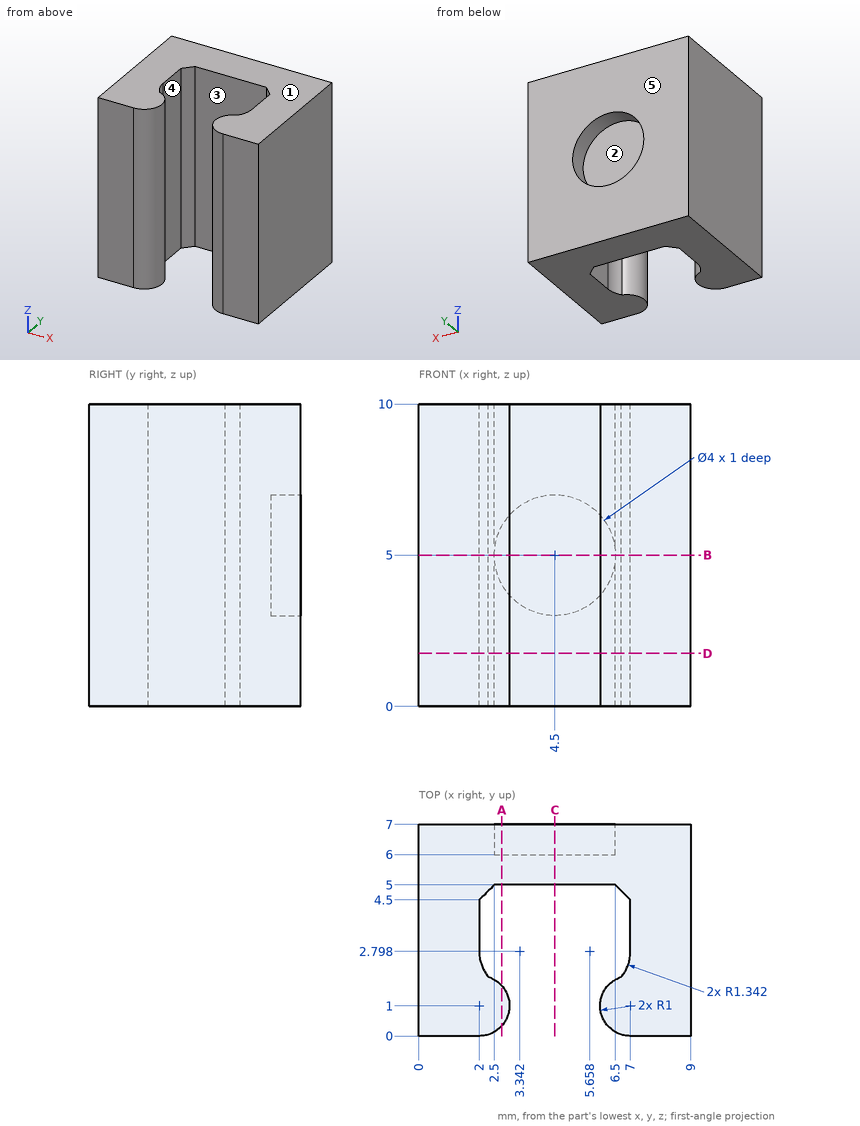
Geometry: see drawing. Coordinates: mm, zero at the bounding-box minimum. A direction names the side the tool comes from. Round coordinates to 2 decimals unless told otherwise and drop trailing zeros. Loops run counter-clockwise (first coordinate to the right, second up) from the corner with the lowest first, then second, coordinate; pieces in that order, holes last. Notation, with made-up numbers: (78.25, 69) -> (103.25, 69) arc R21 cw to (103.25, 74) -> close; hole circle Ø2 at (3, 60). An arc over 180 degrees is marked (long way). Write each question's results on one line, items separated by ' | '.
Item 1: Pull-direction query (Y, two-part tool) for the marked faces 1, 2 and 3; classes: pulls with the +Y half, pulls with the -Y half, needs draft (parallel to the pull), parting line crosses it, or undercut.
Answers below:
face 1: needs draft | face 2: pulls with the +Y half | face 3: undercut
Item 2: Cut plane A-A on x = 2.75. Return the cut outline in (y, z), and give its area (3 significant figures).
Answers below:
outline: (0.34, 0) -> (1.66, 0) -> (1.66, 10) -> (0.34, 10) -> close; (5, 0) -> (7, 0) -> (7, 4.03) -> (6, 4.03) -> (6, 5.97) -> (7, 5.97) -> (7, 10) -> (5, 10) -> close | area: 31.3 mm²
Item 3: Set-up query: the marked faces 4 and 5. Return all of +Z, -Z, +X, -X, +Y, -Y with unobstructed straight access to the full face (end or side cutting, diameter ignored); none if empty.
Answers below:
face 4: +Z, -Z | face 5: +Z, -Z, +X, -X, +Y
Item 4: Cut plane B-B on z = 5. Return the cut outline in (x, y) (1 decimal).
Answers below:
outline: (0, 0) -> (2, 0) arc R1 ccw to (2.3, 2) arc R1.3 cw to (2, 2.8) -> (2, 4.5) -> (2.5, 5) -> (6.5, 5) -> (7, 4.5) -> (7, 2.8) arc R1.3 cw to (6.7, 2) arc R1 ccw to (7, 0) -> (9, 0) -> (9, 7) -> (6.5, 7) -> (6.5, 6) -> (2.5, 6) -> (2.5, 7) -> (0, 7) -> close
Item 5: Cut plane C-C on x = 4.5. Return the cut outline in (y, z).
Answers below:
outline: (5, 0) -> (7, 0) -> (7, 3) -> (6, 3) -> (6, 7) -> (7, 7) -> (7, 10) -> (5, 10) -> close
Item 6: Cut plane D-D on z = 1.75. Return the cut outline in (x, y) (1 decimal).
Answers below:
outline: (0, 0) -> (2, 0) arc R1 ccw to (2.3, 2) arc R1.3 cw to (2, 2.8) -> (2, 4.5) -> (2.5, 5) -> (6.5, 5) -> (7, 4.5) -> (7, 2.8) arc R1.3 cw to (6.7, 2) arc R1 ccw to (7, 0) -> (9, 0) -> (9, 7) -> (0, 7) -> close
Item 7: Line query: probe 1 along X at (y, z) = (2.75, 8.25); probe 2 along Z at (x, y) = (4.5, 6.75); probe 3 along X at (y, z) = (0.75, 7). Output: solid intervals per line, ascending. Write a range as [from, to].
Answers below:
probe 1: x = [0, 2], [7, 9] | probe 2: z = [0, 3], [7, 10] | probe 3: x = [0, 2.97], [6.03, 9]
Item 8: Pin query (flat end, axial travel): pin 1 Ø2 at (x, y) = (5, 3.5) entering from -Z; pin 2 Ø4.5 at (x, z) = (4.5, 5) entering from -Y; pin 3 Ø3 at (x, z) = (4, 5.5) entering from -Y. Return the tip coordinate at first contact, or that it passes through.
Answers below:
pin 1: passes through | pin 2: stops at y = 0.03 | pin 3: stops at y = 0.13
